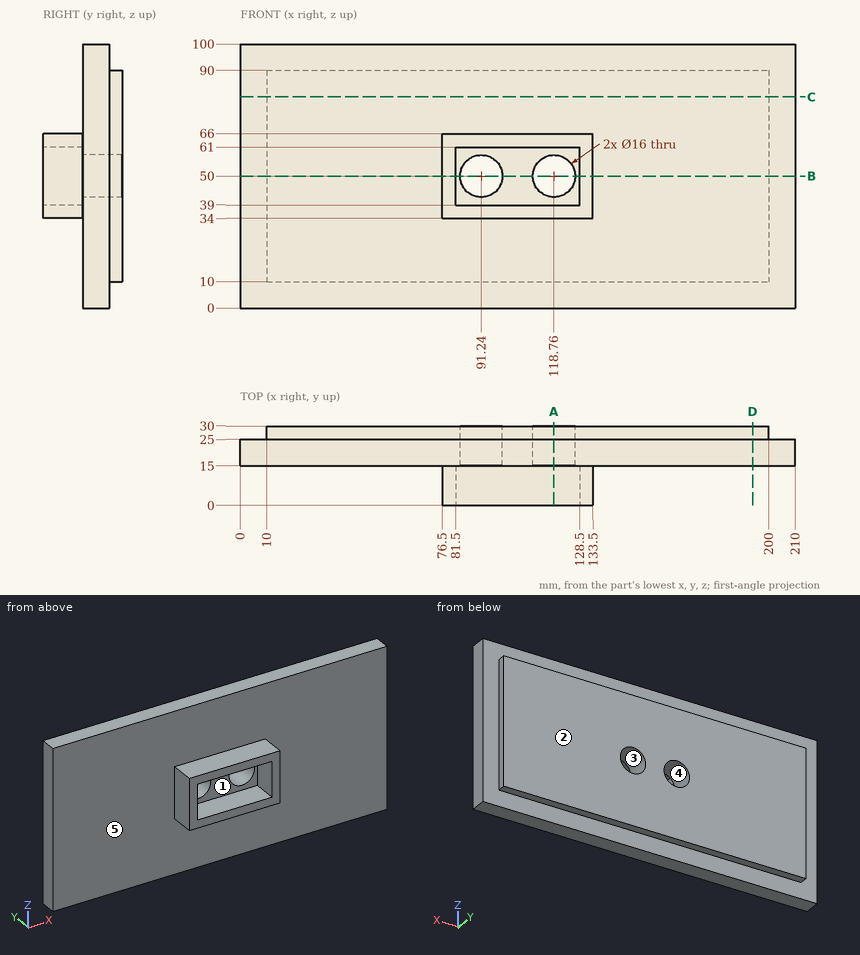
Can you work these out from the drawing? Everything is in mm from the part's minimum corner. A direction names the side the tool comes from. Give positions to 0.01 mm unless a question says otherwise; leave off trailing zeros. Order: outer loops, then holes, each group sorted by start corner. A loop starts at its lowest first (then second) coordinate and runs counter-clockwise, first axis right, second up. Notation, with made-up numbers: M 89.25,51.5 L 131.25,51.5 A35 ccw 131.25,87.5 Z; hole C -13,-16 d6. An arc over 180 degrees is marked long. Use a Markdown table: item, result. Add a question column.
Item 1: Suppose I cut it at A-A (x = 118.76). List the corners of the cut face in (y, z) for me, then the cut area to 3 significant figures.
Item 2: For the marked faces 1 and 2, which set-ups out of +Z, -Z, +X, -X, +Y, -Y let a thin tool reach every point of the face, with its end or its side?
Item 3: Suppose I cut it at D-D (x = 194). List the corners of the cut face in (y, z) for me, then the cut area to 3 significant figures.
Item 4: If I drill on L1, parallel to X at y = 23, z = 50; L2, parallel to X at y = 26.5, z = 50; L3, parallel to Z at x = 91.24, y = 23.25, over which ranges is the centre line in solid material (lowest first)? Write a range as [from, to].
Item 5: Suppose I cut it at B-B (z = 50). List the corners of the cut face in (x, y) for me.
Item 6: We'd pull the mould along Z, two halves only. Please class the marked faces 3, 4 and 5: +Z half, -Z half, draft (parallel to the pull), parting line (faces both ways), or undercut.
Item 7: Suppose I cut it at C-C (z = 80). List the corners of the cut face in (x, y) for me, then the cut area to 3 significant figures.
Item 8: Will these pins go through, and if not, where does the flat tip stop? pin 1 (4.5 mm diameter, centred on y = 10.5, z = 47.5, fed in from -X); pin 2 (14.5 mm diameter, centred on x = 118.76, z = 50, fed in from -Y); pin 3 (4.5 mm diameter, centred on x = 113.5, y = 10.5, fed in from -Z); pin 4 (10 mm diameter, centred on x = 178, z = 20.5, fed in from -Y).
Answer sheet:
| question | item | result |
|---|---|---|
| 1 | outline | M 0,34 L 15,34 L 15,0 L 25,0 L 25,10 L 30,10 L 30,42 L 15,42 L 15,39 L 0,39 Z; M 0,61 L 15,61 L 15,58 L 30,58 L 30,90 L 25,90 L 25,100 L 15,100 L 15,66 L 0,66 Z |
| 1 | area | 1,310 mm² |
| 2 | face 1 | -Y |
| 2 | face 2 | +Z, -Z, +X, -X, +Y |
| 3 | outline | M 15,0 L 25,0 L 25,10 L 30,10 L 30,90 L 25,90 L 25,100 L 15,100 Z |
| 3 | area | 1,400 mm² |
| 4 | L1 | x = [0, 83.24], [99.24, 110.76], [126.76, 210] |
| 4 | L2 | x = [10, 83.24], [99.24, 110.76], [126.76, 200] |
| 4 | L3 | z = [0, 42], [58, 100] |
| 5 | outline | M 0,15 L 76.5,15 L 76.5,0 L 81.5,0 L 81.5,15 L 83.24,15 L 83.24,30 L 10,30 L 10,25 L 0,25 Z; M 99.24,15 L 110.76,15 L 110.76,30 L 99.24,30 Z; M 126.76,15 L 128.5,15 L 128.5,0 L 133.5,0 L 133.5,15 L 210,15 L 210,25 L 200,25 L 200,30 L 126.76,30 Z |
| 6 | face 3 | undercut |
| 6 | face 4 | undercut |
| 6 | face 5 | draft |
| 7 | outline | M 0,15 L 210,15 L 210,25 L 200,25 L 200,30 L 10,30 L 10,25 L 0,25 Z |
| 7 | area | 3,050 mm² |
| 8 | pin 1 | stops at x = 76.5 |
| 8 | pin 2 | passes through |
| 8 | pin 3 | stops at z = 34 |
| 8 | pin 4 | stops at y = 15 |
